Read the model definition and answer for the solid it produces. Units are mm, in the model's axes. A direction names the side the tool comes from. Give positions to 0.01 mm unless a question says otherwise; leave off trailing zeros. Order: outer loops, then holes, each group sorted by start corner. A loop starts at its lowest first (then second) coordinate and runs counter-clockwise, first axis right, second up. Notation, with made-up numbers: M 9,-33 L 33,-33 A21 ccw 33,-7 Z; hole C 68,66.5 d2. An arc over 180 degrees is marked long. One line per item, written item: value. Start each with the question number.
from build123d import *

# Parameters (mm, degrees)
CUT_EXTRUDE_1_DEPTH = 2.58


with BuildPart() as part:
    # Sketch 1 → Revolve 1 (revolve)
    with BuildSketch(Plane.XY):
        with BuildLine():
            Line((0, 2), (-9.435105037, 2))
            ThreePointArc((-9.435105037, 2), (-9.513251262, 2.015899029), (-9.578972997, 2.061068326))
            Line((-9.578972997, 2.061068326), (-11.45137755, 4))
            Line((-11.45137755, 4), (-12, 4))
            Line((-12, 4), (-12, 0))
            Line((-12, 0), (0, 0))
            Line((0, 0), (0, 2))
        make_face()
    revolve(axis=Axis((0, 0, 0), (-1, 0, 0)))

    # Sketch 2 → Cut-Extrude 1 (cut)
    with BuildSketch(Plane.ZY.offset(12)):
        Polygon((0, 1.443375673), (-1.25, 0.721687836), (-1.25, -0.721687836), (0, -1.443375673), (1.25, -0.721687836), (1.25, 0.721687836), align=None)
    extrude(amount=-CUT_EXTRUDE_1_DEPTH, mode=Mode.SUBTRACT)

    # Sketch 6 → Revolve 2 (revolve)
    with BuildSketch(Plane.XY, mode=Mode.PRIVATE) as revolve_2_sk:
        Polygon((-10.5, 1.443375673), (-9.666666667, 0), (-9.05, 0), (-9.05, 1.443375673), align=None)
    revolve(revolve_2_sk.sketch.rotate(Axis((-12, 0, 0), (1, 0, 0)), 90), axis=Axis((-12, 0, 0), (1, 0, 0)))

    # Sketch 7 → Cut-Revolve 2 (revolve, cut)
    with BuildSketch(Plane.XY):
        Polygon((-12, 1.443375673), (-12, 0), (-11.593, 0), align=None)
    revolve(axis=Axis((-12, 0, 0), (1, 0, 0)), mode=Mode.SUBTRACT)

    # Sketch 4 → Cut-Revolve 1 (revolve, cut)
    with BuildSketch(Plane.XY):
        Polygon((-0.35, 2), (0, 1.393782217), (0.35, 2), align=None)
    revolve(axis=Axis((-0.35, 0, 0), (1, 0, 0)), mode=Mode.SUBTRACT)


solid = part.part
Q1. Determine the mould class of faces 1 (the flat face through (0, 0, 0)), 2 (the flat face through (-11, 0, -1.25)), 3 (the conical face through (-9.696, -0.473, 2.13)) for opening direction Z: released by +Z, released by -Z, zero draft, split by the parting line, or undercut.
Q2. A tool of negligible diameter and unlimited length cuts with its end or side. For faces 4 (the flat face through (-11, 0, 1.25)), 5 (the cylindrical face through (-11.73, -0.867, 3.905)), 6 (the cylindrical face through (-5, 0, 2)), from which of +Z, -Z, +X, -X, +Y, -Y can it reach the whole face along a straight path? Write none if from no direction.
Q3. Consider probe 1 along Y at (x, z) = (-7.25, 0); probe 2 along Y at (x, z) = (-10.75, -0.25); probe 3 along X at (y, z) = (1.75, -0.75). Determine where each line is inside the solid, lowest interval first.
Q4. Find section A-A, the plane x = -7.5. Give the vertices of the cut face in (y, z).
Q5. Each of these flat-tipped pins is pushed along its axis until it touches: pin 1 (4 mm diameter, centred on x = -9.5, z = 2.5, fed in from -Y) (3 decimals); pin 2 (1.5 mm diameter, centred on x = -9, z = 3, fed in from +Y) (3 decimals); pin 3 (3 mm diameter, centred on x = -4, z = -1.5, fed in from +Y); pin 4 (0.7 mm diameter, centred on x = -11, y = 0, fed in from -Z) (3 decimals). Where does it stop, or does it pass through?
Evaluation:
1. face 1: zero draft
1. face 2: undercut
1. face 3: split by the parting line
2. face 4: -X
2. face 5: +X, -X
2. face 6: +X
3. probe 1: -2 to 2
3. probe 2: -3.26 to -1.3, 1.3 to 3.26
3. probe 3: -12 to -0.29
4. outline: C 0,0 d4
5. pin 1: y = -3.485
5. pin 2: through
5. pin 3: y = 2
5. pin 4: z = -3.895
